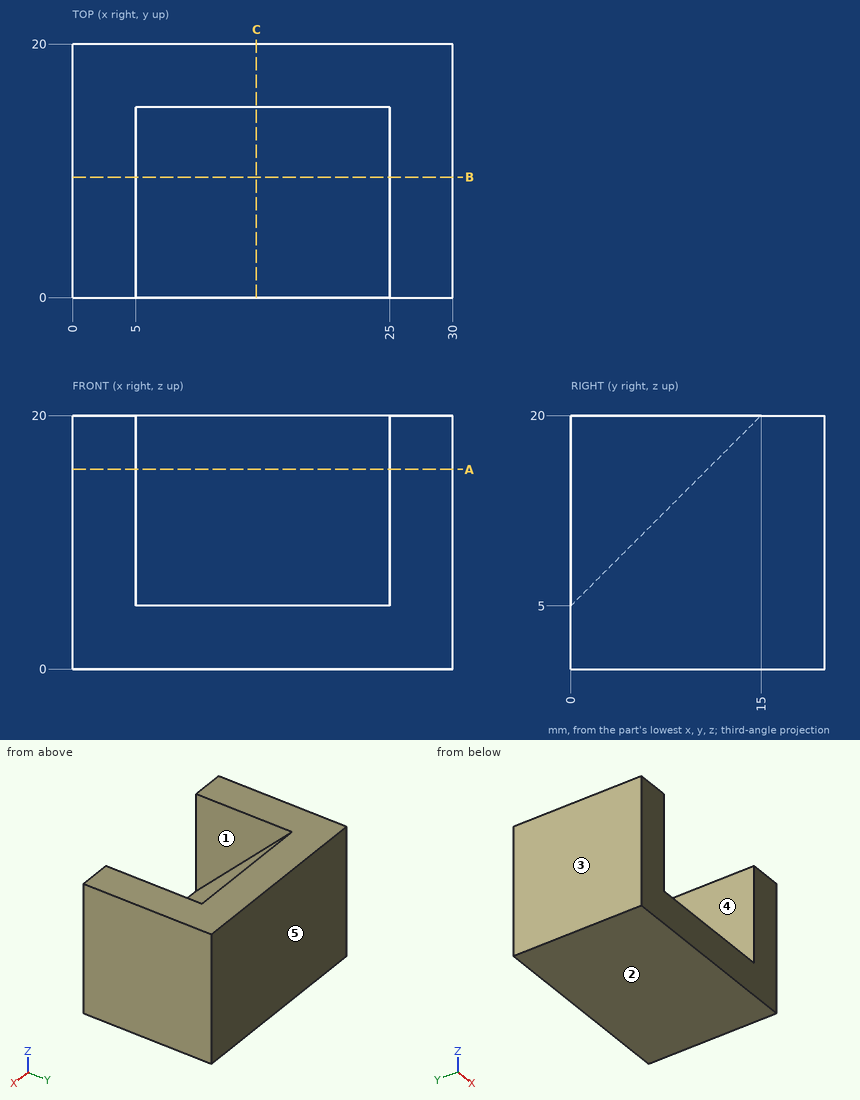
Input: dimensioned drawing with shaded views. Units: mm. Origin: part minimum x, y, z. A direction names the side the tool comes from. Coordinates: 2 decimals unless noted, no trailing zeros. Loops run counter-clockwise (first coordinate to the right, second up) from the corner with the lowest first, then second, coordinate; pieces in that order, holes last. Notation, with made-up numbers: M 76.5,-7 L 131.5,-7 A22 cw 131.5,15 Z; hole C -31.75,73 d10. An arc over 180 degrees is marked long. Use a Markdown table: item, result. Add a question column.
Q1. Draft query along X for the marked faces 1, 2 and 3. Return one class per face: pulls with the +X half, pulls with the -X half, needs draft (parallel to the pull), parting line crosses it, or undercut.
Q2. Access query for the marked faces 4 and 5. Directions: +Z, -Z, +X, -X, +Y, -Y. A direction counts if a zero-diameter tool reaches every point of the face in a straight line with its end or side. Return the directions, or none.
Q3. Section query B-B, the plane y = 9.5. Return loops of the section in (x, z).
Q4. Material intervals for L1, parallel to X at y = 8.25, z = 17; L2, parallel to Y at x = 9.5, z = 18.25; L3, parallel to Z at x = 8.5, y = 11, sorted ascending.
Q5. First-contact query: pin 1 (12 mm diameter, centred on x = 23.5, z = 10, fed in from -Y). Flat tip, straight axial feed; report the tip coordinate or a pass-through.
Q6. Section query A-A, the plane z = 15.75. Return loops of the section in (x, y).
Q7. Section query C-C, the plane x = 14.5. Return loops of the section in (y, z).
Result:
| question | item | result |
|---|---|---|
| 1 | face 1 | undercut |
| 1 | face 2 | needs draft |
| 1 | face 3 | pulls with the -X half |
| 2 | face 4 | +Z, -Y |
| 2 | face 5 | +Z, -Z, +X, -X, +Y |
| 3 | outline | M 0,0 L 30,0 L 30,20 L 25,20 L 25,14.5 L 5,14.5 L 5,20 L 0,20 Z |
| 4 | L1 | x = 0 to 5, 25 to 30 |
| 4 | L2 | y = 13.25 to 20 |
| 4 | L3 | z = 0 to 16 |
| 5 | pin 1 | stops at y = 0 |
| 6 | outline | M 0,0 L 5,0 L 5,10.75 L 25,10.75 L 25,0 L 30,0 L 30,20 L 0,20 Z |
| 7 | outline | M 0,0 L 20,0 L 20,20 L 15,20 L 0,5 Z |
